```python
from build123d import *

# Parameters (mm, degrees)
F0_R     = 69.85
F0_R_2   = 44.45
F1_DEPTH = 22.25
F2_R     = 10
F3_R     = 5
F7_DEPTH = 2
F9_DEPTH = 20


with BuildPart() as f1:
    # F0 (on Front) → F1 (new body, symmetric)
    with BuildSketch(Plane.XZ):
        with Locations((0, 69.85)):
            Circle(F0_R)
        with Locations((0, 69.85)):
            Circle(F0_R_2, mode=Mode.SUBTRACT)
    extrude(amount=F1_DEPTH, both=True)

    # F2
    f2_edges = [f1.edges().sort_by_distance(p)[0] for p in [
        (-69.85, -22.25, 69.85),
        (-69.85, 22.25, 69.85),
    ]]
    fillet(f2_edges, radius=F2_R)

    # F3
    f3_edges = [f1.edges().sort_by_distance(p)[0] for p in [
        (-44.45, 22.25, 69.85),
        (-44.45, -22.25, 69.85),
    ]]
    fillet(f3_edges, radius=F3_R)



with BuildPart() as f7:
    # F5 (on face) → F7 (new body)
    with BuildSketch(Plane(origin=(0, 0, -4.8), x_dir=(1, 0, 0), z_dir=(0, 0, -1))):
        with BuildLine():
            Line((58.9, 10), (58.9, -10))
            Line((58.9, -10), (67.5496086478, -10))
            Line((67.5496086478, -10), (67.5496086478, -2.8))
            Line((67.5496086478, -2.8), (66.7, -2.8))
            ThreePointArc((66.7, -2.8), (63.9, 0), (66.7, 2.8))
            Line((66.7, 2.8), (67.5496086478, 2.8))
            Line((67.5496086478, 2.8), (67.5496086478, 10))
            Line((67.5496086478, 10), (58.9, 10))
        make_face()
        with BuildLine():
            Line((67.5496086478, -2.8), (67.5496086478, -10))
            Line((67.5496086478, -10), (73.3, -10))
            Line((73.3, -10), (77, -6.3))
            Line((77, -6.3), (77, 6.3))
            Line((77, 6.3), (73.3, 10))
            Line((73.3, 10), (67.5496086478, 10))
            Line((67.5496086478, 10), (67.5496086478, 2.8))
            Line((67.5496086478, 2.8), (70.5, 2.8))
            ThreePointArc((70.5, 2.8), (72.4798989873, 1.9798989873), (73.3, 0))
            ThreePointArc((73.3, 0), (72.4798989873, -1.9798989873), (70.5, -2.8))
            Line((70.5, -2.8), (67.5496086478, -2.8))
        make_face()
    extrude(amount=-F7_DEPTH)


with BuildPart() as f7b:
    # F5 (on face) → F7, piece 2 (new body)
    with BuildSketch(Plane(origin=(0, 0, -4.8), x_dir=(1, 0, 0), z_dir=(0, 0, -1))):
        Polygon((-76.8326967955, 6.4673032045), (-76.8326967955, -6.4673032045), (-73.3, -10), (-58.9, -10), (-58.9, 10), (-73.3, 10), align=None)
        with BuildLine():
            ThreePointArc((-70.5, -2.8), (-73.3, 0), (-70.5, 2.8))
            Line((-70.5, 2.8), (-66.7, 2.8))
            ThreePointArc((-66.7, 2.8), (-64.7201010127, 1.9798989873), (-63.9, 0))
            ThreePointArc((-63.9, 0), (-64.7201010127, -1.9798989873), (-66.7, -2.8))
            Line((-66.7, -2.8), (-70.5, -2.8))
        make_face(mode=Mode.SUBTRACT)
    extrude(amount=-F7_DEPTH)


with BuildPart() as f1_1:
    add(f1.part)

    add(f7.part)  # F9 merges F7

    add(f7b.part)  # F9 merges F7b
    # F8 (on face) → F9 (join, through all)
    with BuildSketch(Plane(origin=(0, 10, 0), x_dir=(-1, 0, 0), z_dir=(0, 1, 0))):
        with BuildLine():
            Line((58.9, -2.8), (43.9892310261, 15.5916360942))
            ThreePointArc((43.9892310261, 15.5916360942), (43.4982300473, 15.1972188928), (43.0036928197, 14.8072447649))
            Line((43.0036928197, 14.8072447649), (58.9, -4.8))
            Line((58.9, -4.8), (58.9, -2.8))
        make_face()
        with BuildLine():
            ThreePointArc((-43.0036928197, 14.8072447649), (-43.4982300473, 15.1972188928), (-43.9892310261, 15.5916360942))
            Line((-43.9892310261, 15.5916360942), (-58.9, -2.8))
            Line((-58.9, -2.8), (-58.9, -4.8))
            Line((-58.9, -4.8), (-43.0036928197, 14.8072447649))
        make_face()
    extrude(amount=-F9_DEPTH)


solid = f1_1.part
```
Design review of the part built by this model. Coordinates are the model's own, in mm. A direction names the side the tool comes from. Round coordinates to 2 decimals unless told otherwise and drop trailing zeros. Order: outer loops, then holes, each group sorted by start corner. A loop starts at its lowest first (then second) coordinate and runs counter-clockwise, first axis right, second up. Notation, with made-up numbers: (-2, 33.25) - (20, 33.25) arc R21 cw to (20, 67.25) - close; hole circle Ø8 at (-4, 69.25). An arc over 180 degrees is marked (long way). One line per question, with ' | ' between items.
Item 1: Draft analysis for pull direction Z (two halves, no side actions). For faces 5 (the face through (64, 2, -2.8)), 6 (the face through (-64, 2, -4.8)), 7 (the face through (-75, -8.3, -3.8)), state which applies: +Z half, -Z half, draft (parallel to the pull), parting line (faces both ways), or undercut.
Checks:
face 5: undercut | face 6: -Z half | face 7: draft
Item 2: Take a section at B-B, the plane x = 0. Write out the cut boundary in (y, z).
Checks:
outline: (-22.25, 10) arc R10 ccw to (-12.25, 0) - (12.25, 0) arc R10 ccw to (22.25, 10) - (22.25, 20.4) arc R5 ccw to (17.25, 25.4) - (-17.25, 25.4) arc R5 ccw to (-22.25, 20.4) - close; (-22.25, 119.3) arc R5 ccw to (-17.25, 114.3) - (17.25, 114.3) arc R5 ccw to (22.25, 119.3) - (22.25, 129.7) arc R10 ccw to (12.25, 139.7) - (-12.25, 139.7) arc R10 ccw to (-22.25, 129.7) - close
Item 3: Take a section at A-A, the plane z = 69.85. Write out the cut boundary in (x, y), then the cut area to 3 significant figures.
Checks:
outline: (-69.85, -12.25) arc R10 ccw to (-59.85, -22.25) - (-49.45, -22.25) arc R5 ccw to (-44.45, -17.25) - (-44.45, 17.25) arc R5 ccw to (-49.45, 22.25) - (-59.85, 22.25) arc R10 ccw to (-69.85, 12.25) - close; (44.45, -17.25) arc R5 ccw to (49.45, -22.25) - (59.85, -22.25) arc R10 ccw to (69.85, -12.25) - (69.85, 12.25) arc R10 ccw to (59.85, 22.25) - (49.45, 22.25) arc R5 ccw to (44.45, 17.25) - close | area: 2,150 mm²
Item 4: Machinability: for faces 1 (the face through (51.06, 0.14, 4.87)), 2 (the face through (57, 10, -1)), 3 (the face through (-57, 10, -1)), 4 (the face through (-51.549, 0.14, 6.267)), which of the approach directions +Z, -Z, +X, -X, +Y, -Y give a long, thin tool a straight path to every point of the face, cutting with its end or side? Answer none if there is none.
Checks:
face 1: -Z, +Y, -Y | face 2: -Z, +X, +Y | face 3: -Z, -X, +Y | face 4: -X, +Y, -Y
Item 5: Wall thickness on line 1 (Z direction, x = 0, y = -2); line 2 (X direction, y = 7, z = 69); line 3 (Z direction, x = -5, y = 18.5): over which ranges is each line inside the solid? List them lowest first. Write a range as [from, to].
Checks:
line 1: [0, 25.4], [114.3, 139.7] | line 2: [-69.84, -44.44], [44.44, 69.84] | line 3: [2.38, 25.52], [114.18, 137.32]
Item 6: For P1, Ø1.5, axis at x = -41.5, y = 14.5, coming from the +Z side; P2, Ø2, axis at y = -11.5, z = 113.5, coming from the +X side; P3, Ø12, axis at x = 7, y = 11, coming from the +Z side, all flat-tipped, find the tip position at first contact; note any pin that passes through.
Checks:
P1: z = 126.3 | P2: x = 55.32 | P3: z = 139.69
